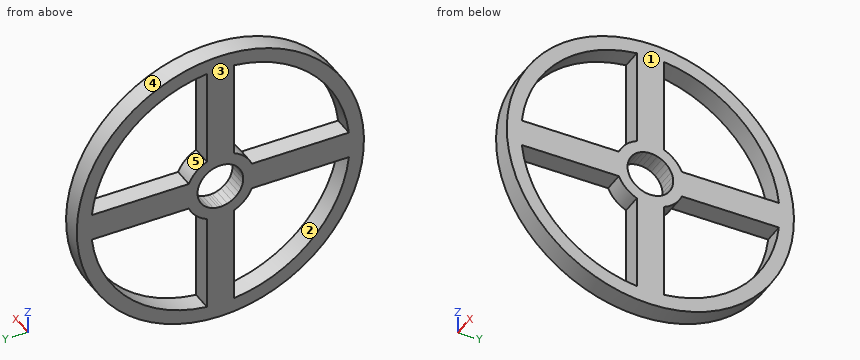
```python
from build123d import *

# Parameters (mm, degrees)
SKETCH3_R           = 50
BOSS_EXTRUDE3_DEPTH = 7


with BuildPart() as part:
    # Sketch3 → Boss-Extrude3 (new body)
    with BuildSketch(Plane(origin=(0, 0, 0), x_dir=(0, 0, -1), z_dir=(1, 0, 0))):
        Circle(SKETCH3_R)
        with BuildLine():
            Line((-4.708862012, -10.983128814), (-4.708862012, -44.752950948))
            ThreePointArc((-4.708862012, -44.752950948), (-31.819805153, -31.819805153), (-44.752950948, -4.708862012))
            Line((-44.752950948, -4.708862012), (-10.983128814, -4.708862012))
            ThreePointArc((-10.983128814, -4.708862012), (-8.449926035, -8.449926035), (-4.708862012, -10.983128814))
        make_face(mode=Mode.SUBTRACT)
        with BuildLine():
            Line((10.983128814, -4.708862012), (44.752950948, -4.708862012))
            ThreePointArc((44.752950948, -4.708862012), (31.819805153, -31.819805153), (4.708862012, -44.752950948))
            Line((4.708862012, -44.752950948), (4.708862012, -10.983128814))
            ThreePointArc((4.708862012, -10.983128814), (8.449926035, -8.449926035), (10.983128814, -4.708862012))
        make_face(mode=Mode.SUBTRACT)
        with BuildLine():
            ThreePointArc((-44.752950948, 4.708862012), (-31.819805153, 31.819805153), (-4.708862012, 44.752950948))
            Line((-4.708862012, 44.752950948), (-4.708862012, 10.983128814))
            ThreePointArc((-4.708862012, 10.983128814), (-8.449926035, 8.449926035), (-10.983128814, 4.708862012))
            Line((-10.983128814, 4.708862012), (-44.752950948, 4.708862012))
        make_face(mode=Mode.SUBTRACT)
        with BuildLine():
            ThreePointArc((-1.652897942, 7.776273426), (-0.831001283, 7.906449068), (0, 7.95))
            ThreePointArc((0, 7.95), (0.831001283, 7.906449068), (1.652897942, 7.776273426))
            ThreePointArc((1.652897942, 7.776273426), (2.456685105, 7.560899305), (3.233556312, 7.262686388))
            ThreePointArc((3.233556312, 7.262686388), (3.975, 6.88490196), (4.672892756, 6.431685105))
            ThreePointArc((4.672892756, 6.431685105), (5.319588321, 5.908001363), (5.908001363, 5.319588321))
            ThreePointArc((5.908001363, 5.319588321), (6.431685105, 4.672892756), (6.88490196, 3.975))
            ThreePointArc((6.88490196, 3.975), (7.262686388, 3.233556312), (7.560899305, 2.456685105))
            ThreePointArc((7.560899305, 2.456685105), (7.776273426, 1.652897942), (7.906449068, 0.831001283))
            ThreePointArc((7.906449068, 0.831001283), (7.939104801, 0.416070852), (7.95, 0))
            ThreePointArc((7.95, 0), (7.939104801, -0.416070852), (7.906449068, -0.831001283))
            ThreePointArc((7.906449068, -0.831001283), (7.776273426, -1.652897942), (7.560899305, -2.456685105))
            ThreePointArc((7.560899305, -2.456685105), (7.262686388, -3.233556312), (6.88490196, -3.975))
            ThreePointArc((6.88490196, -3.975), (6.431685105, -4.672892756), (5.908001363, -5.319588321))
            ThreePointArc((5.908001363, -5.319588321), (5.319588321, -5.908001363), (4.672892756, -6.431685105))
            ThreePointArc((4.672892756, -6.431685105), (3.975, -6.88490196), (3.233556312, -7.262686388))
            ThreePointArc((3.233556312, -7.262686388), (2.456685105, -7.560899305), (1.652897942, -7.776273426))
            ThreePointArc((1.652897942, -7.776273426), (0.831001283, -7.906449068), (0, -7.95))
            ThreePointArc((0, -7.95), (-0.831001283, -7.906449068), (-1.652897942, -7.776273426))
            ThreePointArc((-1.652897942, -7.776273426), (-2.456685105, -7.560899305), (-3.233556312, -7.262686388))
            ThreePointArc((-3.233556312, -7.262686388), (-3.975, -6.88490196), (-4.672892756, -6.431685105))
            ThreePointArc((-4.672892756, -6.431685105), (-5.319588321, -5.908001363), (-5.908001363, -5.319588321))
            ThreePointArc((-5.908001363, -5.319588321), (-6.431685105, -4.672892756), (-6.88490196, -3.975))
            ThreePointArc((-6.88490196, -3.975), (-7.262686388, -3.233556312), (-7.560899305, -2.456685105))
            ThreePointArc((-7.560899305, -2.456685105), (-7.776273426, -1.652897942), (-7.906449068, -0.831001283))
            ThreePointArc((-7.906449068, -0.831001283), (-7.95, 0), (-7.906449068, 0.831001283))
            ThreePointArc((-7.906449068, 0.831001283), (-7.776273426, 1.652897942), (-7.560899305, 2.456685105))
            ThreePointArc((-7.560899305, 2.456685105), (-7.262686388, 3.233556312), (-6.88490196, 3.975))
            ThreePointArc((-6.88490196, 3.975), (-6.431685105, 4.672892756), (-5.908001363, 5.319588321))
            ThreePointArc((-5.908001363, 5.319588321), (-5.319588321, 5.908001363), (-4.672892756, 6.431685105))
            ThreePointArc((-4.672892756, 6.431685105), (-3.975, 6.88490196), (-3.233556312, 7.262686388))
            ThreePointArc((-3.233556312, 7.262686388), (-2.456685105, 7.560899305), (-1.652897942, 7.776273426))
        make_face(mode=Mode.SUBTRACT)
        with BuildLine():
            Line((4.708862012, 10.983128814), (4.708862012, 44.752950948))
            ThreePointArc((4.708862012, 44.752950948), (31.819805153, 31.819805153), (44.752950948, 4.708862012))
            Line((44.752950948, 4.708862012), (10.983128814, 4.708862012))
            ThreePointArc((10.983128814, 4.708862012), (8.449926035, 8.449926035), (4.708862012, 10.983128814))
        make_face(mode=Mode.SUBTRACT)
    extrude(amount=BOSS_EXTRUDE3_DEPTH)


solid = part.part
```
CAD build for the part. Positions are in the model's coordinates, mm. Face numbers are marked on the shaded views. A direction names the side the tool comes from. Round coordinates to 2 decimals unless told otherwise and drop trailing zeros. Write each loop counter-clockwise with the first axis right and the second up, starting at its lowest first coordinate (ties: lowest second). Pieces come first, ordered by that corner, then holes. Notation, with made-up numbers: (71.25, 26) - (89.25, 26) arc R25 cw to (89.25, 50) - close; hole circle Ø2 at (41, -28). An arc over 180 degrees is marked (long way). Return JSON: item names as keys, results as strings. Group by question number.
Item 1: Band-saw the part on C-C on x = 4.5. List the corners of the cut face in (y, z) (3 decimals).
Item 2: Probe probe 1 along Z at (x, y) = (1.25, 13.5); probe 2 along Y at (x, z) = (0.75, -6.5); probe 3 along Y at (x, z) = (6, -20.5). List the from-to ranges inside material, lowest first.
Item 3: Mould opens along Y. For the marked faces 3, 4 and 5 say: +Y half, -Y half, draft (parallel to the pull), parting line (faces both ways), or undercut.
Item 4: Flat gauge pins, fed straight in: pin 1 Ø4 at (x, z) = (2.5, 12.5) entering from -Y; pin 2 Ø3.5 at (x, z) = (2, 23.5) entering from -Y; pin 3 Ø2 at (x, z) = (5, -24) entering from -Y. Where does each tip first touch, or does it go through?
Item 5: 3-axis set-ups, long thin cutter, end or side, ignore diameter. For the marked faces 1 and 2: which of +Z, -Z, +X, -X, +Y, -Y reach the whole face in a straight line?
Item 6: Band-saw the part on B-B on y = 35. List the corners of the cut face in (x, z).
Item 7: Band-saw the part on A-A on z = -18. List the corners of the cut face in (x, y).
Resolved:
{
 "1": {"outline": "circle Ø100 at (0, 0); hole (-44.753, -4.709) arc R45 ccw to (-4.709, -44.753) - (-4.709, -10.983) arc R11.95 cw to (-10.983, -4.709) - close; hole (-44.753, 4.709) - (-10.983, 4.709) arc R11.95 cw to (-4.709, 10.983) - (-4.709, 44.753) arc R45 ccw to start; hole circle Ø15.9 at (0, 0); hole (4.709, -44.753) arc R45 ccw to (44.753, -4.709) - (10.983, -4.709) arc R11.95 cw to (4.709, -10.983) - close; hole (4.709, 10.983) arc R11.95 cw to (10.983, 4.709) - (44.753, 4.709) arc R45 ccw to (4.709, 44.753) - close"},
 "2": {"probe 1": "z = -48.14 to -42.93, -4.71 to 4.71, 42.93 to 48.14", "probe 2": "y = -49.58 to -44.53, -10.03 to -4.58, 4.58 to 10.03, 44.53 to 49.58", "probe 3": "y = -45.6 to -40.06, -4.71 to 4.71, 40.06 to 45.6"},
 "3": {"face 3": "draft", "face 4": "parting line", "face 5": "undercut"},
 "4": {"pin 1": "stops at y = -48.89", "pin 2": "stops at y = -45.02", "pin 3": "stops at y = -44.4"},
 "5": {"face 1": "+Z, -Z, +X, +Y, -Y", "face 2": "+X, -X"},
 "6": {"outline": "(0, -35.71) - (7, -35.71) - (7, -28.28) - (0, -28.28) - close; (0, -4.71) - (7, -4.71) - (7, 4.71) - (0, 4.71) - close; (0, 28.28) - (7, 28.28) - (7, 35.71) - (0, 35.71) - close"},
 "7": {"outline": "(0, -46.65) - (7, -46.65) - (7, -41.24) - (0, -41.24) - close; (0, -4.71) - (7, -4.71) - (7, 4.71) - (0, 4.71) - close; (0, 41.24) - (7, 41.24) - (7, 46.65) - (0, 46.65) - close"}
}
